from build123d import *

# Parameters (mm, degrees)
BOSS_EXTRUDE1_DEPTH = 45.72
SHELL1_T            = 2.54


with BuildPart() as part:
    # Sketch7 → Boss-Extrude1 (new body)
    with BuildSketch(Plane.XY):
        Polygon((9.655091904, 152.134877954), (82.143686264, 152.134877954), (82.143686264, -4.447468667), (14.497027414, -4.447468667), (3.305091904, -4.447468667), (3.305091904, 92.914044904), (3.305091904, 152.134877954), align=None)
    extrude(amount=BOSS_EXTRUDE1_DEPTH)

    # Shell1
    shell1_openings = [part.faces().sort_by_distance(p)[0] for p in [
        (42.724389084, 73.843704643, 45.72),
    ]]
    offset(amount=SHELL1_T, openings=shell1_openings, kind=Kind.INTERSECTION)


solid = part.part
Build history of the part. All positions in model axes, mm. A direction names the side the tool comes from. Round coordinates to 2 decimals unless told otherwise and drop trailing zeros. Write each loop counter-clockwise with the first axis right and the second up, starting at its lowest first coordinate (ties: lowest second). Pieces come first, ordered by that corner, then holes. Notation, with made-up numbers: M 88,77.5 L 125,77.5 A28 cw 125,114.5 Z; hole C 5.5,46.25 d8. An arc over 180 degrees is marked long. Answer as a JSON object with one key per item and string values. Group by question number.
(1) Cut at B-B (x = 7). Give the cut face in (y, z), and give its area (3 significant figures).
(2) Flat gauge pin, fed straight in: pin 1 (1 mm diameter, centred on x = 43, y = 71.5, fed in from +Z). Where does the tip first touch, or does it go through?
(3) Drill centre lines: L1, parallel to Y at x = 20.5, z = 16; L2, parallel to X at y = 15.5, z = 25.5; L3, parallel to Z at x = 37.5, y = 109. Where is each one in solid material? Low to high.
(4) Which spindle directions (+Z, -Z, +X, -X, +Y, -Y) get a long thin tool onto all of the face, cutting with end or side? Do faces 1 (the flat face through (3, 74, 45.72)), 2 (the flat face through (43, 152.135, 23)). Say none if no direction does.
(5) Cut at A-A (z = 8). Give the cut face in (x, y).
(6) Cut at C-C (y = 113). Give the cut face in (x, z).
(7) Mould opens along X. For faces 3 (the flat face through (3.305, 75, 23)), 4 (the flat face through (0.765, 75, 21)), 5 (the flat face through (43, 154.675, 21)) say: pulls with the +X half, pulls with the -X half, needs draft (parallel to the pull), parting line crosses it, or undercut.
Responses:
{
 "1": {"outline": "M -6.99,-2.54 L 154.67,-2.54 L 154.67,45.72 L 152.13,45.72 L 152.13,0 L -4.45,0 L -4.45,45.72 L -6.99,45.72 Z", "area": "643 mm2"},
 "2": {"pin 1": "stops at z = 0"},
 "3": {"L1": "y = -6.99 to -4.45, 152.13 to 154.67", "L2": "x = 0.77 to 3.31, 82.14 to 84.68", "L3": "z = -2.54 to 0"},
 "4": {"face 1": "+Z, +X, -X, +Y, -Y", "face 2": "+Z"},
 "5": {"outline": "M 0.77,-6.99 L 84.68,-6.99 L 84.68,154.67 L 0.77,154.67 Z; hole M 3.31,-4.45 L 82.14,-4.45 L 82.14,152.13 L 3.31,152.13 Z"},
 "6": {"outline": "M 0.77,-2.54 L 84.68,-2.54 L 84.68,45.72 L 82.14,45.72 L 82.14,0 L 3.31,0 L 3.31,45.72 L 0.77,45.72 Z"},
 "7": {"face 3": "undercut", "face 4": "pulls with the -X half", "face 5": "needs draft"}
}
